Here's how the part is built. I have some questions about the finished solid (model axes, mm). A direction names the side the tool comes from. Round coordinates to 2 decimals unless told otherwise and drop trailing zeros. Loops run counter-clockwise (first coordinate to the right, second up) from the corner with the lowest first, then second, coordinate; pieces in that order, holes last. Notation, with made-up numbers: M 30,-28.5 L 49,-28.5 A25 cw 49,9.5 Z; hole C 21,-3 d4. An arc over 180 degrees is marked long. Use a Markdown table: item, result.
from build123d import *

# Parameters (mm, degrees)
SKETCH1_R               = 1.95
BOSS_EXTRUDE1_DEPTH     = 50
SKETCH2_W               = 3.9
SKETCH2_H               = 6.4
SKETCH2_H_2             = 4
CUT_EXTRUDE1_DEPTH      = 51.075992252
CUT_EXTRUDE2_DEPTH      = 51.075992252
CUT_EXTRUDE2_DEPTH_BACK = 51.075992252
SKETCH3_W               = 0.4
SKETCH3_H               = 6.4
CUT_EXTRUDE3_DEPTH      = 51.075992252
CUT_EXTRUDE3_DEPTH_BACK = 51.075992252
SKETCH4_R               = 1.35
SKETCH5_R               = 1.235
CUT_EXTRUDE4_DEPTH      = 51.075992359
BOSS_EXTRUDE2_DEPTH     = 1
CUT_EXTRUDE5_DEPTH      = 97.039601311


with BuildPart() as part:
    # Sketch1 → Boss-Extrude1 (new, symmetric)
    with BuildSketch(Plane(origin=(0, 0, 0), x_dir=(1, 0, 0), z_dir=(0, 1, 0))):
        with Locations(Location((0, 0, 0), (0, 0, 270))):
            Circle(SKETCH1_R)
    extrude(amount=BOSS_EXTRUDE1_DEPTH, both=True)

    # Sketch2 → Cut-Extrude1 (cut, through all)
    with BuildSketch(Plane.XY):
        with Locations((0, -46.8)):
            Rectangle(SKETCH2_W, SKETCH2_H)
        with Locations((0, 48)):
            Rectangle(SKETCH2_W, SKETCH2_H_2)
    extrude(amount=-CUT_EXTRUDE1_DEPTH, mode=Mode.SUBTRACT)

    # Sketch3 → Cut-Extrude2 (cut, two sides: drawn at the far end of the back side and taken through both)
    with BuildSketch(Plane(origin=(0, 0, 0), x_dir=(0, 0, -1), z_dir=(1, 0, 0)).offset(-CUT_EXTRUDE2_DEPTH_BACK)):
        with Locations((-1.75, -46.8)):
            Rectangle(SKETCH3_W, SKETCH3_H)
    extrude(amount=CUT_EXTRUDE2_DEPTH + CUT_EXTRUDE2_DEPTH_BACK, mode=Mode.SUBTRACT)

    # Sketch4 → Cut-Extrude3 (cut, two sides: drawn at the far end of the back side and taken through both)
    with BuildSketch(Plane(origin=(0, 0, 0), x_dir=(-1, 0, 0), z_dir=(0, 0, -1)).offset(-CUT_EXTRUDE3_DEPTH_BACK)):
        with Locations((0, -46.6)):
            Circle(SKETCH4_R)
    extrude(amount=CUT_EXTRUDE3_DEPTH + CUT_EXTRUDE3_DEPTH_BACK, mode=Mode.SUBTRACT)

    # Sketch5 → Cut-Extrude4 (cut, through all)
    with BuildSketch(Plane(origin=(0, 0, 0), x_dir=(-1, 0, 0), z_dir=(0, 0, -1))):
        with Locations((0, 45.89)):
            Circle(SKETCH5_R)
    extrude(amount=CUT_EXTRUDE4_DEPTH, mode=Mode.SUBTRACT)

    # Sketch6 → Boss-Extrude2 (add)
    with BuildSketch(Plane(origin=(0, 0, 0), x_dir=(-1, 0, 0), z_dir=(0, 0, -1))):
        with BuildLine():
            Line((-1.95, 46), (-1.23009146, 46))
            ThreePointArc((-1.23009146, 46), (0, 47.125), (1.23009146, 46))
            Line((1.23009146, 46), (1.95, 46))
            Line((1.95, 46), (1.95, 50))
            Line((1.95, 50), (-1.95, 50))
            Line((-1.95, 50), (-1.95, 46))
        make_face()
    extrude(amount=BOSS_EXTRUDE2_DEPTH)

    # Sketch7 → Cut-Extrude5 (cut, through all)
    with BuildSketch(Plane.XZ.offset(-46)):
        with BuildLine():
            Line((1.95, -1), (1.95, 0))
            ThreePointArc((1.95, 0), (1.879751375, -0.518685616), (1.674066904, -1))
            Line((1.674066904, -1), (1.95, -1))
        make_face()
        with BuildLine():
            Line((-1.95, -1), (-1.674066904, -1))
            ThreePointArc((-1.674066904, -1), (-1.879751375, -0.518685616), (-1.95, 0))
            Line((-1.95, 0), (-1.95, -1))
        make_face()
    extrude(amount=-CUT_EXTRUDE5_DEPTH, mode=Mode.SUBTRACT)


solid = part.part
1. For pin 1 Ø1.2 at (x, y) = (0, -45) entering from +Z; pin 2 Ø1.5 at (x, y) = (1, -1) entering from +Z; pin 3 Ø1.5 at (x, y) = (0.5, -28.5) entering from -Z; pin 4 Ø1.6 at (x, y) = (0, -46.6) entering from +Z, each with a flat end and sliding along its axis, tell me the tip position at first contact or that it passes through.
Answer sheet:
| item | result |
|---|---|
| pin 1 | z = 1.55 |
| pin 2 | z = 1.93 |
| pin 3 | z = -1.95 |
| pin 4 | through |
2. Imagine slicing it at C-C, the plane y = -38. Write out the boundary of the cut face in (x, z).
Answer sheet:
| item | result |
|---|---|
| outline | C 0,0 d3.9 |
3. Imagine slicing it at B-B, the plane z = 0.8. Write out the boundary of the cut face in (x, y).
Answer sheet:
| item | result |
|---|---|
| outline | M -1.78,-50 L 1.78,-50 L 1.78,50 L -1.78,50 Z; hole C 0,-46.6 d2.7 |
4. I need wall thicknesses on probe 1 along X at (y, z) = (-34.5, 0.15); probe 2 along X at (y, z) = (-46.6, 0.5); probe 3 along X at (y, z) = (-46.6, 1). Which ranges of each line are inside material? Lowest first, please. Write a range as from..to.
Answer sheet:
| item | result |
|---|---|
| probe 1 | -1.94..1.94 |
| probe 2 | -1.88..-1.35, 1.35..1.88 |
| probe 3 | -1.67..-1.35, 1.35..1.67 |
5. We'd pull the mould along X, two halves only. Please class faces 1 (the face through (0.29, -47.92, 0.79)), 2 (the face through (0, -49, 1.55)): +X half, -X half, draft (parallel to the pull), parting line (faces both ways), or undercut.
Answer sheet:
| item | result |
|---|---|
| face 1 | undercut |
| face 2 | draft |
6. Which directions (+Z, -Z, +X, -X, +Y, -Y) give clear straight access to the entire face, cutting with the end or side of a thin tool? Please do faces 3 (the face through (0, 48, -1)), 4 (the face through (0, 46, 0)), 5 (the face through (0, -45, 1.55)), 6 (the face through (0, -48.2, 0)).
Answer sheet:
| item | result |
|---|---|
| face 3 | -Z, +X, -X, +Y |
| face 4 | -Z |
| face 5 | +Z, +X, -X, -Y |
| face 6 | -Z, +X, -X, -Y |
7. Imagine slicing it at A-A, the plane x = 0. Write out the boundary of the cut face in (y, z) (3 decimals), then the cut area to 3 significant figures.
Answer sheet:
| item | result |
|---|---|
| outline | M -50,0 L -47.95,0 L -47.95,1.55 L -50,1.55 Z; M -45.25,0 L -43.6,0 L -43.6,-1.95 L 44.655,-1.95 L 44.655,0 L 47.125,0 L 47.125,-1 L 50,-1 L 50,1.95 L -43.6,1.95 L -43.6,1.55 L -45.25,1.55 Z |
| area | 363 mm2 |
